Geometry check sheet. Reference: the model listing, model coordinates, mm. Face numbers are marked on the shaded views. A direction names the side the tool comes from. Give positions to 0.01 mm unless a question says otherwise; leave off trailing zeros. Write each loop counter-clockwise with the first axis right and the second up, starting at its lowest first coordinate (ties: lowest second). Pieces come first, ordered by that corner, then holes. Notation, with made-up numbers: (8, -37) -> (13, -37) arc R27 ccw to (13, 0) -> close; hole circle Ø8 at (-38.5, 7). An arc over 180 degrees is marked (long way). Use a Markdown table: item, result. Add a question column.
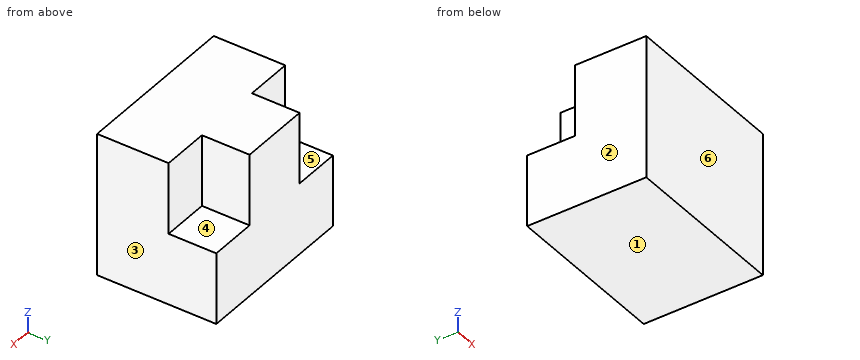
from build123d import *

# Parameters (mm, degrees)
SKETCH1_W           = 35
SKETCH1_H           = 25
BOSS_EXTRUDE1_DEPTH = 15
BOSS_EXTRUDE2_DEPTH = 15


with BuildPart() as part:
    # Sketch1 → Boss-Extrude1 (new body)
    with BuildSketch(Plane.XY):
        with Locations((-5.777889773, 0.039936102)):
            Rectangle(SKETCH1_W, SKETCH1_H)
    extrude(amount=-BOSS_EXTRUDE1_DEPTH)

    # Sketch2 → Boss-Extrude2 (add)
    with BuildSketch(Plane.XY):
        Polygon((-13.277889773, 12.539936102), (1.722110227, 12.539936102), (1.722110227, 2.539936102), (11.722110227, 2.539936102), (11.722110227, -12.460063898), (-23.277889773, -12.460063898), (-23.277889773, 2.539936102), (-13.277889773, 2.539936102), align=None)
    extrude(amount=BOSS_EXTRUDE2_DEPTH)


solid = part.part
1) Sectioned sample at C-C, the plane y = 4.75. Enter the section's corners in (x, z), and give its area (3 significant figures).
2) Sectioned sample at B-B, the plane x = -16. Enter the section's corners in (y, z).
3) Material ranges on probe 1 along Y at (x, z) = (2, 0.5); probe 2 along Z at (x, y) = (-14, 10.5), recorded low to high. Write a range as [from, to].
4) Sectioned sample at A-A, the plane z = 5.5. Enter the section's corners in (x, y), and give its area (3 significant figures).
5) Draft check along X on the marked faces 1, 2 and 3. Enter one of: +X half, -X half, draft (parallel to the pull), parting line (faces both ways), or undercut.
6) Gauge pin test, flat ends, axial feed: P1, Ø8, axis at x = -17.5, y = 9, coming from the +Z side; P2, Ø4, axis at x = -16, z = 4.5, coming from the +Y side; P3, Ø8, axis at y = 9.5, z = 11, coming from the -X side. Record the tip position at first contact, or that the pin passes through.
7) Tool access check on the marked faces 4, 5 and 6. Record the directions out of +Z, -Z, +X, -X, +Y, -Y that give a thin tool (end or side, any length) a straight path to the whole face; none if there is none.
Check values:
| question | item | result |
|---|---|---|
| 1 | outline | (-23.28, -15) -> (11.72, -15) -> (11.72, 0) -> (1.72, 0) -> (1.72, 15) -> (-13.28, 15) -> (-13.28, 0) -> (-23.28, 0) -> close |
| 1 | area | 750 mm² |
| 2 | outline | (-12.46, -15) -> (12.54, -15) -> (12.54, 0) -> (2.54, 0) -> (2.54, 15) -> (-12.46, 15) -> close |
| 3 | probe 1 | [-12.46, 2.54] |
| 3 | probe 2 | [-15, 0] |
| 4 | outline | (-23.28, -12.46) -> (11.72, -12.46) -> (11.72, 2.54) -> (1.72, 2.54) -> (1.72, 12.54) -> (-13.28, 12.54) -> (-13.28, 2.54) -> (-23.28, 2.54) -> close |
| 4 | area | 675 mm² |
| 5 | face 1 | draft |
| 5 | face 2 | -X half |
| 5 | face 3 | +X half |
| 6 | P1 | z = 0 |
| 6 | P2 | y = 2.54 |
| 6 | P3 | x = -13.28 |
| 7 | face 4 | +Z, +X, +Y |
| 7 | face 5 | +Z, -X, +Y |
| 7 | face 6 | +Z, -Z, +X, -X, -Y |
